```python
from build123d import *

# Parameters (mm, degrees)
SKETCH1_R           = 1.4
BOSS_EXTRUDE1_DEPTH = 3


with BuildPart() as part:
    # Sketch1 → Boss-Extrude1 (new body)
    with BuildSketch(Plane(origin=(0, 0, 0), x_dir=(1, 0, 0), z_dir=(0, 1, 0))):
        with BuildLine():
            Line((66.715956662, -50.018199395), (23.228889619, -6.531132352))
            ThreePointArc((23.228889619, -6.531132352), (16.157821807, -6.531132352), (16.157821807, -13.602200164))
            Line((16.157821807, -13.602200164), (59.64488885, -57.089267207))
            ThreePointArc((59.64488885, -57.089267207), (59.937782069, -57.796373988), (59.64488885, -58.503480769))
            Line((59.64488885, -58.503480769), (53.63448121, -64.513888409))
            ThreePointArc((53.63448121, -64.513888409), (52.755801554, -66.635208753), (53.63448121, -68.756529097))
            Line((53.63448121, -68.756529097), (59.998442241, -75.120490127))
            ThreePointArc((59.998442241, -75.120490127), (62.119762584, -75.999169784), (64.241082928, -75.120490127))
            Line((64.241082928, -75.120490127), (70.251490568, -69.110082487))
            ThreePointArc((70.251490568, -69.110082487), (70.958597349, -68.817189268), (71.665704131, -69.110082487))
            Line((71.665704131, -69.110082487), (98.535761816, -95.980140172))
            ThreePointArc((98.535761816, -95.980140172), (99.242868597, -96.273033391), (99.949975378, -95.980140172))
            Line((99.949975378, -95.980140172), (105.606829627, -90.323285923))
            ThreePointArc((105.606829627, -90.323285923), (105.899722846, -89.616179142), (105.606829627, -88.90907236))
            Line((105.606829627, -88.90907236), (78.736771942, -62.039014675))
            ThreePointArc((78.736771942, -62.039014675), (78.443878724, -61.331907894), (78.736771942, -60.624801113))
            Line((78.736771942, -60.624801113), (84.747179582, -54.614393473))
            ThreePointArc((84.747179582, -54.614393473), (85.625859239, -52.493073129), (84.747179582, -50.371752786))
            Line((84.747179582, -50.371752786), (78.383218552, -44.007791755))
            ThreePointArc((78.383218552, -44.007791755), (76.261898208, -43.129112099), (74.140577865, -44.007791755))
            Line((74.140577865, -44.007791755), (68.130170225, -50.018199395))
            ThreePointArc((68.130170225, -50.018199395), (67.423063443, -50.311092614), (66.715956662, -50.018199395))
        make_face()
        with Locations((19.693355713, -10.066666258)):
            Circle(SKETCH1_R, mode=Mode.SUBTRACT)
        with BuildLine():
            Line((82.625859239, -70.87784944), (100.303528769, -88.55551897))
            ThreePointArc((100.303528769, -88.55551897), (100.303528769, -90.676839313), (98.182208425, -90.676839313))
            Line((98.182208425, -90.676839313), (80.504538895, -72.999169784))
            ThreePointArc((80.504538895, -72.999169784), (80.504538895, -70.87784944), (82.625859239, -70.87784944))
        make_face(mode=Mode.SUBTRACT)
        with BuildLine():
            Line((60.7762597, -65.99881265), (75.625502105, -51.149570245))
            ThreePointArc((75.625502105, -51.149570245), (77.605401092, -51.149570245), (77.605401092, -53.129469232))
            Line((77.605401092, -53.129469232), (62.756158688, -67.978711637))
            ThreePointArc((62.756158688, -67.978711637), (60.7762597, -67.978711637), (60.7762597, -65.99881265))
        make_face(mode=Mode.SUBTRACT)
        with BuildLine():
            Line((27.825083697, -16.077073898), (57.877121897, -46.129112099))
            ThreePointArc((57.877121897, -46.129112099), (57.877121897, -48.250432442), (55.755801554, -48.250432442))
            Line((55.755801554, -48.250432442), (25.703763353, -18.198394242))
            ThreePointArc((25.703763353, -18.198394242), (25.703763353, -16.077073898), (27.825083697, -16.077073898))
        make_face(mode=Mode.SUBTRACT)
    extrude(amount=BOSS_EXTRUDE1_DEPTH)


solid = part.part
```
Input: part model. Units: mm. Frame: model coordinates. A direction names the side the tool comes from. Give positions to 0.01 mm unless a question says otherwise; leave off trailing zeros. Order: outer loops, then holes, each group sorted by start corner. A loop starts at its lowest first (then second) coordinate and runs counter-clockwise, first axis right, second up. Notation, with made-up numbers: M 56.5,64 L 64.5,64 A19 ccw 64.5,94 Z; hole C -37.5,35 d8. An arc over 180 degrees is marked long. One line per question, with ' | ' between items. Start each with the question number.
1. Material intervals for probe 1 along X at (y, z) = (2.05, 72); probe 2 along Z at (x, y) = (48, 0.95); probe 3 along Z at (x, y) = (73.5, 2), sorted ascending. Write a range as [from, to].
2. Section query C-C (y = 2.55). Count the separate pieces of the cut face and the enclosed holes in it, and give its area (3 significant figures).
3. Access query for faces 4 (the face through (56.68, 1.48, 61.47)), 5 (the face through (84.913, 1.479, 82.357)), 6 (the face through (68.097, 1.479, 58.678)), 7 (the face through (71.18, 1.48, 46.97)), 8 (the face through (60, 3, 54)). Directions: +Z, -Z, +X, -X, +Y, -Y. A direction counts if a zero-diameter tool reaches every point of the face in a straight line with its end or side. Return the directions, or none.
4. Section query B-B (z = 31). Return the cut outline in (x, y), and give its area (3 significant figures).
5. Section query A-A (x = 29). Return the cut outline in (y, z), and give its area (3 significant figures).
6. First-contact query: pin 1 Ø5 at (x, z) = (92, 81) entering from -Y; pin 2 Ø1.5 at (y, z) = (1.5, 58.5) entering from -X; pin 3 Ø1.5 at (y, z) = (2.5, 18) entering from +X; pin 4 Ø2 at (x, z) = (19.69, 10.07) entering from +Y. Flat tips, straight axial feed; report the tip coordinate or a pass-through.
7. Pull-direction query (Z, two-part tool) for faces 1 (the face through (67.2, 1.48, 72.16)), 2 (the face through (81.61, 1.479, 47.234)), 3 (the face through (91.34, 1.48, 79.59)); classes: released by +Z, released by -Z, zero draft, split by the parting line, or undercut.
Here are the results:
1) probe 1: [56.88, 67.36], [74.56, 80.07], [83.75, 88.7] | probe 2: [31.3, 36.25], [40.49, 45.44] | probe 3: [44.65, 53.28], [57.23, 70.94]
2) separate pieces: 1 | enclosed holes: 4 | area: 1,290 mm²
3) face 4: -X, +Y, -Y | face 5: +Z, +Y, -Y | face 6: +Y, -Y | face 7: -Z, +Y, -Y | face 8: +Z, -Z, +X, -X, +Y
4) outline: M 33.56,0 L 38.51,0 L 38.51,3 L 33.56,3 Z; M 42.75,0 L 47.7,0 L 47.7,3 L 42.75,3 Z | area: 29.7 mm²
5) outline: M 0,12.3 L 3,12.3 L 3,17.25 L 0,17.25 Z; M 0,21.49 L 3,21.49 L 3,26.44 L 0,26.44 Z | area: 29.7 mm²
6) pin 1: y = 0 | pin 2: x = 58.9 | pin 3: x = 35.45 | pin 4: through
7) face 1: released by +Z | face 2: released by -Z | face 3: undercut
